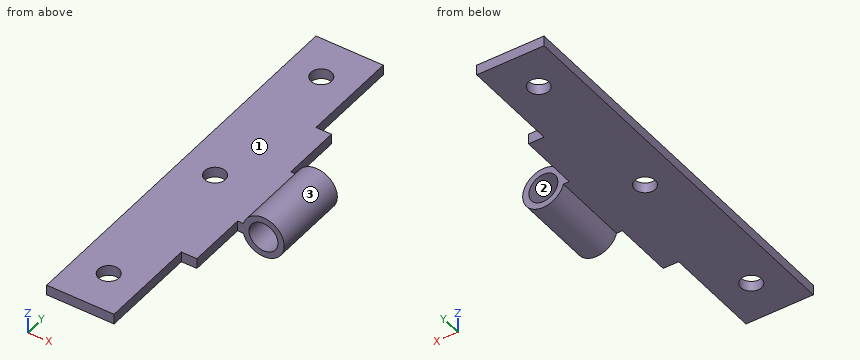
```python
from build123d import *

# Parameters (mm, degrees)
SKETCH1_R           = 1.4
BOSS_EXTRUDE1_DEPTH = 7.5
SKETCH2_W           = 8
SKETCH2_H           = 1
BOSS_EXTRUDE2_DEPTH = 5.75
SKETCH3_W           = 8
SKETCH3_H           = 1
BOSS_EXTRUDE3_DEPTH = 5.75
SKETCH4_W           = 6.5
SKETCH4_H           = 1
BOSS_EXTRUDE4_DEPTH = 9.5
SKETCH5_W           = 6.5
SKETCH5_H           = 1
BOSS_EXTRUDE5_DEPTH = 9.5
CUT_EXTRUDE1_REACH  = 4.5
SKETCH6_R           = 1


with BuildPart() as part:
    # Sketch1 → Boss-Extrude1 (new body)
    with BuildSketch(Plane(origin=(0, 0, 0), x_dir=(1, 0, 0), z_dir=(0, 1, 0))):
        with BuildLine():
            Line((2.313508327, 0.5), (-6.25, 0.5))
            Line((-6.25, 0.5), (-6.25, -0.5))
            Line((-6.25, -0.5), (2.313508327, -0.5))
            ThreePointArc((2.313508327, -0.5), (6.25, 0), (2.313508327, 0.5))
        make_face()
        with Locations((4.25, 0)):
            Circle(SKETCH1_R, mode=Mode.SUBTRACT)
    extrude(amount=BOSS_EXTRUDE1_DEPTH)

    # Sketch2 → Boss-Extrude2 (add)
    with BuildSketch(Plane(origin=(0, 7.5, 0), x_dir=(1, 0, 0), z_dir=(0, 1, 0))):
        with Locations((-2.25, 0)):
            Rectangle(SKETCH2_W, SKETCH2_H)
    extrude(amount=BOSS_EXTRUDE2_DEPTH)

    # Sketch3 → Boss-Extrude3 (add)
    with BuildSketch(Plane.XZ):
        with Locations((-2.25, 0)):
            Rectangle(SKETCH3_W, SKETCH3_H)
    extrude(amount=BOSS_EXTRUDE3_DEPTH)

    # Sketch4 → Boss-Extrude4 (add)
    with BuildSketch(Plane.XZ.offset(5.75)):
        with Locations((-3, 0)):
            Rectangle(SKETCH4_W, SKETCH4_H)
    extrude(amount=BOSS_EXTRUDE4_DEPTH)

    # Sketch5 → Boss-Extrude5 (add)
    with BuildSketch(Plane(origin=(0, 13.25, 0), x_dir=(1, 0, 0), z_dir=(0, 1, 0))):
        with Locations((-3, 0)):
            Rectangle(SKETCH5_W, SKETCH5_H)
    extrude(amount=BOSS_EXTRUDE5_DEPTH)

    # Sketch6 → Cut-Extrude1 (cut, up to next)
    with BuildSketch(Plane.XY.offset(0.5), mode=Mode.PRIVATE) as cut_extrude1_sk1:
        with Locations((-3, 18.75)):
            Circle(SKETCH6_R)
    cut_extrude1_tool1 = extrude(cut_extrude1_sk1.sketch, amount=-CUT_EXTRUDE1_REACH, mode=Mode.PRIVATE) & part.part
    add(cut_extrude1_tool1.solids().sort_by_distance((-3, 18.75, 0.5))[0], mode=Mode.SUBTRACT)
    # Sketch6 → Cut-Extrude1 (cut, up to next)
    with BuildSketch(Plane.XY.offset(0.5), mode=Mode.PRIVATE) as cut_extrude1_sk2:
        with Locations((-3, 3.75)):
            Circle(SKETCH6_R)
    cut_extrude1_tool2 = extrude(cut_extrude1_sk2.sketch, amount=-CUT_EXTRUDE1_REACH, mode=Mode.PRIVATE) & part.part
    add(cut_extrude1_tool2.solids().sort_by_distance((-3, 3.75, 0.5))[0], mode=Mode.SUBTRACT)
    # Sketch6 → Cut-Extrude1 (cut, up to next)
    with BuildSketch(Plane.XY.offset(0.5), mode=Mode.PRIVATE) as cut_extrude1_sk3:
        with Locations((-3, -11.25)):
            Circle(SKETCH6_R)
    cut_extrude1_tool3 = extrude(cut_extrude1_sk3.sketch, amount=-CUT_EXTRUDE1_REACH, mode=Mode.PRIVATE) & part.part
    add(cut_extrude1_tool3.solids().sort_by_distance((-3, -11.25, 0.5))[0], mode=Mode.SUBTRACT)


solid = part.part
```
For this review, take the finished solid that the model builds, in its own axes (mm). Face numbers are marked on the shaded views. Coordinates: 2 decimals unless noted, no trailing zeros. Loops run counter-clockwise (first coordinate to the right, second up) from the corner with the lowest first, then second, coordinate; pieces in that order, holes last. Notation, with made-up numbers: (54, 54) - (112, 54) arc R25 ccw to (112, 79) - close; hole circle Ø7 at (57, 54). An arc over 180 degrees is marked (long way). Use one line per item in the form item = value. Start each with the question number.
1) Take a section at A-A (z = 0). State the section outline as (x, y) points.
2) To check wall thickness, follow probe 1 along Y at (x, z) = (-3, 0); probe 2 along Z at (x, y) = (4.25, 4.25); probe 3 along Z at (x, y) = (-3, 6.5). State the ranges of each line that lie inside material, in increasing order. Write a range as from..to.
3) Take a section at B-B (y = -11.25). State the section outline as (x, z) points, plus the area to 3 significant figures.
4) Take a section at C-C (x = -3). State the section outline as (y, z) points, plus the area to 3 significant figures.
5) Draft analysis for pull direction X (two halves, no side actions). For the marked faces 1, 2 and 3, state which applies: released by +X, released by -X, zero draft, split by the parting line, or undercut.
6) For pin 1 (4.5 mm diameter, centred on x = -3.5, y = -5, fed in from -Z); pin 2 (2 mm diameter, centred on x = 4.5, z = 0.5, fed in from -Y); pin 3 (2 mm diameter, centred on x = 1, y = 10.5, fed in from +Z), all flat-tipped, find the tip position at first contact; note any pin that passes through.
7) Take a section at D-D (y = 3.75). State the section outline as (x, z) points.
From the geometry:
q1.outline = (-6.25, -15.25) - (0.25, -15.25) - (0.25, -5.75) - (1.75, -5.75) - (1.75, 0) - (2.85, 0) - (2.85, 7.5) - (1.75, 7.5) - (1.75, 13.25) - (0.25, 13.25) - (0.25, 22.75) - (-6.25, 22.75) - close; (5.65, 0) - (6.25, 0) - (6.25, 7.5) - (5.65, 7.5) - close; hole circle Ø2 at (-3, -11.25); hole circle Ø2 at (-3, 3.75); hole circle Ø2 at (-3, 18.75)
q2.probe_1 = -15.25..-12.25, -10.25..2.75, 4.75..17.75, 19.75..22.75
q2.probe_2 = -2..-1.4, 1.4..2
q2.probe_3 = -0.5..0.5
q3.outline = (-6.25, -0.5) - (-4, -0.5) - (-4, 0.5) - (-6.25, 0.5) - close; (-2, -0.5) - (0.25, -0.5) - (0.25, 0.5) - (-2, 0.5) - close
q3.area = 4.50 mm2
q4.outline = (-15.25, -0.5) - (-12.25, -0.5) - (-12.25, 0.5) - (-15.25, 0.5) - close; (-10.25, -0.5) - (2.75, -0.5) - (2.75, 0.5) - (-10.25, 0.5) - close; (4.75, -0.5) - (17.75, -0.5) - (17.75, 0.5) - (4.75, 0.5) - close; (19.75, -0.5) - (22.75, -0.5) - (22.75, 0.5) - (19.75, 0.5) - close
q4.area = 32.0 mm2
q5.face_1 = zero draft
q5.face_2 = undercut
q5.face_3 = split by the parting line
q6.pin_1 = -0.5
q6.pin_2 = 0
q6.pin_3 = 0.5
q7.outline = (-6.25, -0.5) - (-4, -0.5) - (-4, 0.5) - (-6.25, 0.5) - close; (-2, -0.5) - (2.31, -0.5) arc R2 ccw (long way) to (2.31, 0.5) - (-2, 0.5) - close; hole circle Ø2.8 at (4.25, 0)
